from build123d import *

# Parameters (mm, degrees)
F0_R     = 7.5
F1_DEPTH = 35
F2_W     = 3.71815
F2_H     = 12.979131
F3_DEPTH = 12.5
F4_R     = 2.5
F5_DEPTH = 25


with BuildPart() as f1:
    # F0 (on Front) → F1 (new body)
    with BuildSketch(Plane.XZ):
        Circle(F0_R)
    extrude(amount=F1_DEPTH)

    # F2 (on Top) → F3 (cut, symmetric)
    with BuildSketch(Plane.XY):
        with Locations((0, -23.489568)):
            Rectangle(F2_W, F2_H)
    extrude(amount=F3_DEPTH, both=True, mode=Mode.SUBTRACT)

    # F4 (on face) → F5 (cut)
    with BuildSketch(Plane(origin=(0, 0, 0), x_dir=(-1, 0, 0), z_dir=(0, 1, 0))):
        Circle(F4_R)
    extrude(amount=-F5_DEPTH, mode=Mode.SUBTRACT)


solid = f1.part
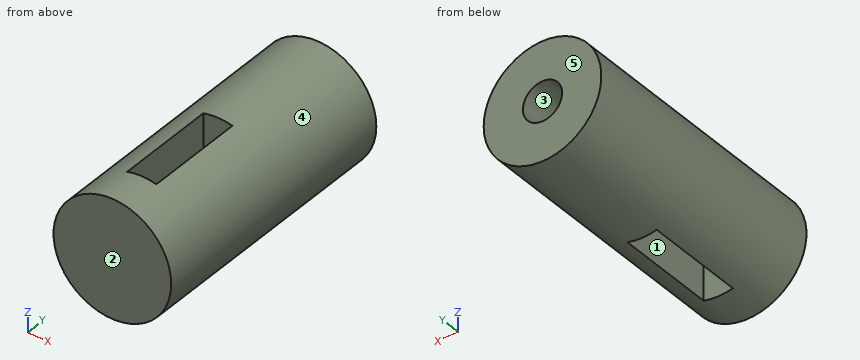
Can you work these out from the model? Positions are in its coordinate system, mm. Face numbers are marked on the shaded views. A direction names the side the tool comes from. Coordinates: 2 decimals unless noted, no trailing zeros. Order: outer loops, then holes, each group sorted by start corner. A loop starts at its lowest first (then second) coordinate and runs counter-clockwise, first axis right, second up. Notation, with made-up numbers: (35, -2.75) - (51, -2.75) arc R13 cw to (51, 1.25) - close; hole circle Ø3 at (-25.75, 53). An arc over 180 degrees is marked (long way). Answer as a JSON object with one key per item and string values. Group by question number.
Q1. Imagine slicing it at C-C (z = 0). Please give me the cut outline in (x, y).
Q2. On a 3-axis mill with a long thin cutter (end or side, diameter ignored), from which of +Z, -Z, +X, -X, +Y, -Y can I reach the whole of each face in a straight line? I mean the marked faces 1 and 2. Say none if no direction works.
Q3. We'd pull the mould along X, two halves only. Please class the marked faces 3, 4 and 5: +X half, -X half, draft (parallel to the pull), parting line (faces both ways), or undercut.
Q4. I need wall thicknesses on line 1 (Y direction, x = -1.5, z = -2.5); line 2 (Z direction, x = 0, y = -14.25); line 3 (X direction, y = -24, z = 2.5). Which ranges of each line are inside material? Lowest first, please. Write a range as from..to.
Q5. Imagine slicing it at D-D (z = 6.75). Please give me the cut outline in (x, y), and give its area (3 significant figures).
Q6. Imagine slicing it at A-A (y = -18). Please give me the cut outline in (x, z).
Q7. Will these pins go through, and if not, where does the flat tip stop? P1, Ø0.7, axis at x = -2, z = 0, coming from the +Y side; P2, Ø5, axis at y = -9.5, z = 3, coming from the +X side; P3, Ø4, axis at y = -5, z = 5, coming from the -X side.
Q8. Imagine slicing it at B-B (x = 0). Please give me the cut outline in (y, z), and give its area (3 significant figures).
Determined:
{
 "1": {"outline": "(-7.5, -35) - (7.5, -35) - (7.5, 0) - (2.5, 0) - (2.5, -25) - (1.86, -25) - (1.86, -29.98) - (-1.86, -29.98) - (-1.86, -25) - (-2.5, -25) - (-2.5, 0) - (-7.5, 0) - close"},
 "2": {"face 1": "+Z, -Z", "face 2": "+Z, -Z, +X, -X, -Y"},
 "3": {"face 3": "undercut", "face 4": "parting line", "face 5": "draft"},
 "4": {"line 1": "y = -35..-29.98, -17..0", "line 2": "z = -7.5..-2.5, 2.5..7.5", "line 3": "x = -7.07..-1.86, 1.86..7.07"},
 "5": {"outline": "(-3.27, -35) - (3.27, -35) - (3.27, 0) - (-3.27, 0) - close; hole (-1.86, -29.98) - (1.86, -29.98) - (1.86, -17) - (-1.86, -17) - close", "area": "181 mm2"},
 "6": {"outline": "(-1.86, -7.27) - (-1.86, -1.67) arc R2.5 cw to (-1.86, 1.67) - (-1.86, 7.27) arc R7.5 ccw to start; (1.86, -7.27) arc R7.5 ccw to (1.86, 7.27) - (1.86, 1.67) arc R2.5 cw to (1.86, -1.67) - close"},
 "7": {"P1": "stops at y = -25", "P2": "stops at x = 7.48", "P3": "stops at x = -6.87"},
 "8": {"outline": "(-35, -7.5) - (-29.98, -7.5) - (-29.98, 7.5) - (-35, 7.5) - close; (-17, -7.5) - (0, -7.5) - (0, -2.5) - (-17, -2.5) - close; (-17, 2.5) - (0, 2.5) - (0, 7.5) - (-17, 7.5) - close", "area": "245 mm2"}
}
